Geometry: see drawing. Coordinates: mm, zero at the bounding-box minimum. Coordinates: 2 decimals unless noted, no trailing zeros. Write each loop counter-clockwise with the first axis right and the second up, starting at its lowest first coordinate (ties: lowest second). Pieces come first, ordered by that corner, then holes.
1) Pin query (flat end, axial travel): pin 1 Ø6 at (y, z) = (18.5, 33.5) entering from +X; pin 2 Ø1 at (y, z) = (36.5, 43) entering from +X; pin 3 Ø2 at (x, y) = (17, 49.5) entering from -Z; pin 4 Ø8 at (x, z) = (15, 61.5) entering from +Y. Return the tip coordinate at first contact, or that it passes through.
2) Line query: L1, parallel to X at y = 31, z = 20; L2, parallel to Y at x = 31.75, z = 21.5; L3, parallel to X at y = 23, z = 60 (1 decimal). Output: solid intervals per line, ascending.
3) Section query A-A (x = 31.75). Output: boundary loops of the cut face in (y, z), then the cut area to 3 significant figures.
4) Draft query along Y for the marked faces 1, 2 and 3. Return one class per face: pulls with the +Y half, pulls with the -Y half, needs draft (parallel to the pull), parting line crosses it, or undercut.
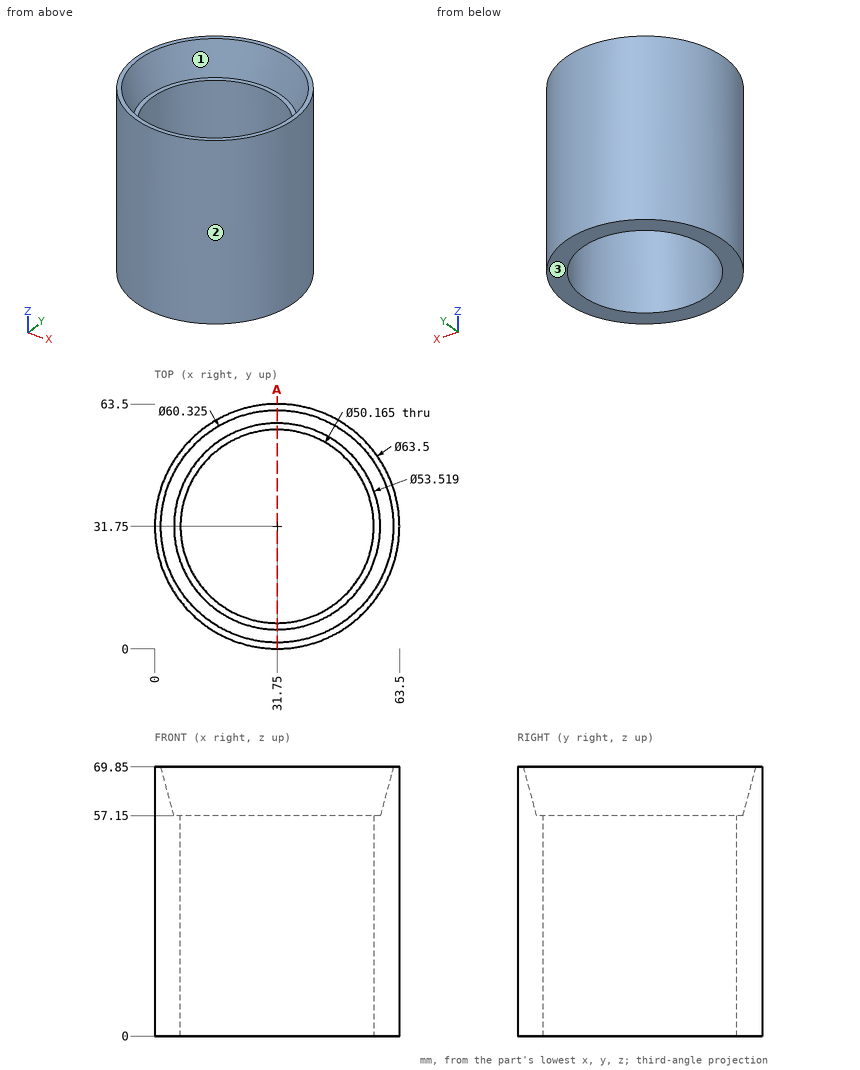
Answer:
1. pin 1: stops at x = 61.8
1. pin 2: stops at x = 63.21
1. pin 3: passes through
1. pin 4: stops at y = 60.83
2. L1: x = 0.01 to 6.68, 56.82 to 63.49
2. L2: y = 0 to 6.67, 56.83 to 63.5
2. L3: x = 1.2 to 5.7, 57.8 to 62.3
3. outline: (0, 0) - (6.67, 0) - (6.67, 57.15) - (4.99, 57.15) - (1.59, 69.85) - (0, 69.85) - close; (56.83, 0) - (63.5, 0) - (63.5, 69.85) - (61.91, 69.85) - (58.51, 57.15) - (56.83, 57.15) - close
3. area: 846 mm2
4. face 1: undercut
4. face 2: parting line crosses it
4. face 3: needs draft
